Autodesk Inventor part; units mm, degrees
ref_plane "YZ Plane" through (0, 0, 0) normal (1, 0, 0) x (0, 1, 0)
ref_plane "XZ Plane" through (0, 0, 0) normal (0, 1, 0) x (-1, 0, 0)
ref_plane "XY Plane" through (0, 0, 0) normal (0, 0, 1) x (1, 0, 0)
sketch "Boceto1" plane through (0, 0, 0) normal (0, 1, 0) x (-1, 0, 0)
  line L0 (0, 0) -> (80, 0)
  line L1 (80, 0) -> (80, -80)
  line L2 (80, -80) -> (0, -80)
  line L3 (0, -80) -> (0, 0)
  line L4 (10, -70) -> (70, -70)
  line L5 (70, -70) -> (70, -10)
  line L6 (70, -10) -> (10, -10)
  line L7 (10, -10) -> (10, -70)
  line L8 (0, -12.375) -> (80, -12.375)
  line L9 (0, -14.95) -> (80, -14.95)
  line L10 (0, -17.525) -> (80, -17.525)
  line L11 (80, -20.1) -> (0, -20.1)
  line L12 (0, -22.675) -> (80, -22.675)
  line L13 (0, -12.575) -> (80, -12.575)
  line L14 (0, -15.15) -> (80, -15.15)
  line L15 (0, -17.725) -> (80, -17.725)
  line L16 (80, -20.3) -> (0, -20.3)
  line L17 (0, -22.875) -> (80, -22.875)
  line L18 (0, -25.25) -> (80, -25.25)
  line L19 (0, -25.45) -> (80, -25.45)
  line L20 (10, -40) -> (80, -40)
  line L21 (0, -67.625) -> (80, -67.625)
  line L22 (0, -65.05) -> (80, -65.05)
  line L23 (0, -62.475) -> (80, -62.475)
  line L24 (80, -59.9) -> (0, -59.9)
  line L25 (0, -57.325) -> (80, -57.325)
  line L26 (0, -67.425) -> (80, -67.425)
  line L27 (0, -64.85) -> (80, -64.85)
  line L28 (0, -62.275) -> (80, -62.275)
  line L29 (80, -59.7) -> (0, -59.7)
  line L30 (0, -57.125) -> (80, -57.125)
  line L31 (0, -54.75) -> (80, -54.75)
  line L32 (0, -54.55) -> (80, -54.55)
  line L33 (75, -5) -> (5, -5)
  line L34 (5, -5) -> (5, -75)
  line L35 (5, -75) -> (75, -75)
  line L36 (75, -75) -> (75, -5)
  line L37 (5, 0) -> (0, 0)
  line L38 (5, -80) -> (0, -80)
  point P0 (10, -12.375)
  point P1 (70, -12.375)
  point P2 (10, -14.95)
  point P3 (70, -14.95)
  point P4 (10, -17.525)
  point P5 (70, -17.525)
  point P6 (70, -20.1)
  point P7 (10, -20.1)
  point P8 (10, -22.675)
  point P9 (70, -22.675)
  point P10 (10, -12.575)
  point P11 (70, -12.575)
  point P12 (10, -15.15)
  point P13 (70, -15.15)
  point P14 (10, -17.725)
  point P15 (70, -17.725)
  point P16 (70, -20.3)
  point P17 (10, -20.3)
  point P18 (10, -22.875)
  point P19 (70, -22.875)
  point P20 (10, -25.25)
  point P21 (70, -25.25)
  point P22 (10, -25.45)
  point P23 (70, -25.45)
  point P24 (10, -67.625)
  point P25 (70, -67.625)
  point P26 (10, -65.05)
  point P27 (70, -65.05)
  point P28 (10, -62.475)
  point P29 (70, -62.475)
  point P30 (70, -59.9)
  point P31 (10, -59.9)
  point P32 (10, -57.325)
  point P33 (70, -57.325)
  point P34 (10, -67.425)
  point P35 (70, -67.425)
  point P36 (10, -64.85)
  point P37 (70, -64.85)
  point P38 (10, -62.275)
  point P39 (70, -62.275)
  point P40 (70, -59.7)
  point P41 (10, -59.7)
  point P42 (10, -57.125)
  point P43 (70, -57.125)
  point P44 (10, -54.75)
  point P45 (70, -54.75)
  point P46 (10, -54.55)
  point P47 (70, -54.55)
  point P48 (75, -12.375)
  point P49 (5, -12.375)
  point P50 (75, -54.55)
  point P51 (75, -25.45)
  point P52 (70, -25.45)
  point P53 (70, -54.55)
  point P54 (5, -25.45)
  point P55 (5, -54.55)
  point P56 (10, -54.55)
  point P57 (10, -25.45)
  point P58 (10, -67.625)
  point P59 (5, -67.625)
  point P60 (75, -67.625)
  point P61 (70, -67.625)
  dimension "d0" = 80
  dimension "d1" = 80
  dimension "d2" = 60
  dimension "d3" = 60
  dimension "d4" = 10
  dimension "d5" = 10
  dimension "d6" = 2.375
  dimension "d7" = 0.2
  dimension "d8" = 2.375
  dimension "d9" = 0.2
  dimension "d10" = 0.2
  dimension "d11" = 0.2
  dimension "d12" = 0.2
  dimension "d13" = 2.375
  dimension "d14" = 2.375
  dimension "d15" = 2.375
  dimension "d16" = 2.375
  dimension "d17" = 0.2
  dimension "d26" = 5
extrude "Extrusión1" add sketch "Boceto1" along normal blind 5 contours L0 L1 L8 L36 L33 L34 L3 | L13 L34 L9 L3 | L34 L33 L36 L8 L5 L6 L7 | L13 L7 L9 L34 | L7 L6 L5 L8 | L1 L9 L36 L13 | L14 L34 L10 L3 | L13 L5 L9 L7 | L36 L9 L5 L13 | L14 L7 L10 L34 | L1 L10 L36 L14 | L15 L34 L11 L3 | L14 L5 L10 L7 | L36 L10 L5 L14 | L15 L7 L11 L34 | L1 L11 L36 L15 | L16 L34 L12 L3 | L15 L5 L11 L7 | L36 L11 L5 L15 | L16 L7 L12 L34 | L1 L12 L36 L16 | L17 L34 L18 L3 | L16 L5 L12 L7 | L36 L12 L5 L16 | L17 L7 L18 L34 | L1 L18 L36 L17 | L19 L34 L32 L3 | L17 L5 L18 L7 | L36 L18 L5 L17 | L19 L7 L32 L34 | L1 L20 L36 L19 | L31 L34 L30 L3 | L19 L5 L20 L7 | L1 L32 L36 L20 | L36 L20 L5 L19 | L31 L7 L30 L34 | L7 L20 L5 L32 | L36 L32 L5 L20 | L25 L34 L29 L3 | L31 L5 L30 L7 | L1 L30 L36 L31 | L25 L7 L29 L34 | L31 L36 L30 L5 | L24 L34 L28 L3 | L25 L5 L29 L7 | L1 L29 L36 L25 | L24 L7 L28 L34 | L25 L36 L29 L5 | L23 L34 L27 L3 | L24 L5 L28 L7 | L1 L28 L36 L24 | L23 L7 L27 L34 | L24 L36 L28 L5 | L22 L34 L26 L3 | L23 L5 L27 L7 | L1 L27 L36 L23 | L22 L7 L26 L34 | L23 L36 L27 L5 | L21 L34 L35 L36 L1 L2 L3 | L22 L5 L26 L7 | L1 L26 L36 L22 | L21 L7 L4 L5 L36 L35 L34 | L22 L36 L26 L5 | L21 L5 L4 L7
sketch "Boceto2" plane through (0, 0, 0) normal (0, -1, 0) x (1, 0, 0)
  line L0 (0, -80) -> (-80, -80)
  line L1 (-80, 0) -> (0, 0)
  line L2 (-80, -80) -> (-80, 0)
  line L3 (-80, 0) -> (0, 0)
  line L4 (-80, -65.05) -> (0, -65.05) construction
  line L5 (0, 0) -> (0, -80)
  line L6 (-80, -80) -> (0, -80)
extrude "Extrusión4" add sketch "Boceto2" along normal blind 3
extrude "Extrusión5" add sketch "Boceto1" along normal blind 10 contours L34 L33 L36 L8 L5 L6 L7 | L19 L7 L32 L34 | L36 L20 L5 L19 | L36 L32 L5 L20 | L21 L7 L4 L5 L36 L35 L34
sketch "Boceto3" plane through (0, 10, 0) normal (0, 1, 0) x (1, 0, 0)
  line L0 (-5, 25.45) -> (-5, 54.55)
  line L1 (-5, 40) -> (-84.1767, 40)
  line L2 (-5, 39.5) -> (-84.1767, 39.5)
  line L3 (-5, 40.5) -> (-84.1767, 40.5)
  line L4 (-10, 54.55) -> (-10, 25.45)
  line L5 (-5, 40.5) -> (-5, 39.5)
  line L6 (-84.1767, 40.5) -> (-84.1767, 39.5)
  point P0 (0, 0)
  point P1 (-10, 40)
  point P2 (-10, 39.5)
  point P3 (-10, 40.5)
  dimension "d31" = 0.5
  dimension "d32" = 0.5
extrude "Extrusión6" cut sketch "Boceto3" against normal blind 2
equation "\"d8\" = d6"
equation "\"d9\" = d7"
equation "\"d10\" = d9"
equation "\"d11\" = d7"
equation "\"d12\" = d7"
equation "\"d13\" = d6"
equation "\"d14\" = d6"
equation "\"d15\" = d6"
equation "\"d16\" = d6"
equation "\"d17\" = d7"
properties part number "Cortador Ancho PDMS"
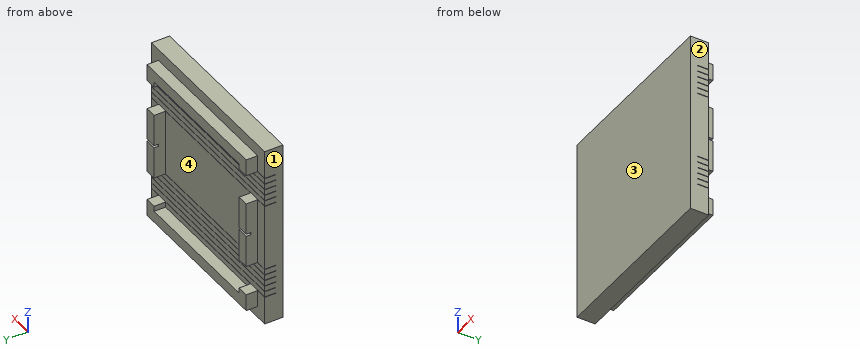
Work out the finished part from the listing and answer in its coordinate system (mm). Face numbers are marked on the shaded views. Give positions to 0.01 mm unless a question says otherwise; leave off trailing zeros. Order: outer loops, then holes, each group sorted by start corner. A loop starts at its lowest first (then second) coordinate and runs counter-clockwise, first axis right, second up. Notation, with made-up numbers: (33, 49.25) -> (58, 49.25) arc R12 cw to (58, 70.25) -> close; hole circle Ø1 at (88.5, -27.75). An arc over 180 degrees is marked (long way). Answer as a JSON object with one key per item and string values. Group by question number.
1. Section B-B on z = -6 is taken. Determine the outline of the cut face in (x, y), plus the area to 3 significant figures.
2. Consider line 1 along Z through (x, y) = (-6.5, 9.75) (3 decimals); line 2 along X through (y, z) = (8.25, -37). Determine where each line is inside the solid, lowest interval first. Write a range as [from, to].
3. The mould has two halves that part along X. Classify the marked faces 1, 2, 3 and 4: released by +X, released by -X, zero draft, split by the parting line, or undercut.
4. Flat-ended cylindrical pins translate along their axes: pin 1 Ø5.5 at (x, y) = (-32, 8.5) entering from -Z; pin 2 Ø0.7 at (y, z) = (7, -69) entering from -X; pin 3 Ø4 at (y, z) = (5.5, -57.5) entering from -X; pin 4 Ø1.5 at (x, z) = (-1.5, -39) entering from +Y. Find the tip coordinate at first contact, or state that the pin passes through.
5. Section A-A on y = 6.25 is taken. Determine the outline of the cut face in (x, z) (3 decimals).
6. Section C-C on y = 1.5 is taken. Count the separate pieces of the cut face and the enclosed holes in it, plus the area to 3 significant figures.
Result sheet:
{
 "1": {"outline": "(-80, -3) -> (0, -3) -> (0, 5) -> (-5, 5) -> (-5, 10) -> (-75, 10) -> (-75, 5) -> (-80, 5) -> close", "area": "990 mm^2"},
 "2": {"line 1": "z = [-75, -67.625], [-54.55, -40.5], [-39.5, -25.45], [-12.375, -5]", "line 2": "x = [-75, -70], [-10, -5]"},
 "3": {"face 1": "released by -X", "face 2": "released by +X", "face 3": "zero draft", "face 4": "undercut"},
 "4": {"pin 1": "stops at z = -75", "pin 2": "stops at x = -75", "pin 3": "stops at x = -80", "pin 4": "stops at y = 5"},
 "5": {"outline": "(-75, -75) -> (-5, -75) -> (-5, -67.625) -> (-10, -67.625) -> (-10, -70) -> (-70, -70) -> (-70, -67.625) -> (-75, -67.625) -> close; (-75, -54.55) -> (-70, -54.55) -> (-70, -25.45) -> (-75, -25.45) -> close; (-75, -12.375) -> (-70, -12.375) -> (-70, -10) -> (-10, -10) -> (-10, -12.375) -> (-5, -12.375) -> (-5, -5) -> (-75, -5) -> close; (-10, -54.55) -> (-5, -54.55) -> (-5, -25.45) -> (-10, -25.45) -> close"},
 "6": {"separate pieces": "13", "enclosed holes": "0", "area": "6,210 mm^2"}
}
